Verification items for the finished model (mm, model axes). A direction names the side the tool comes from. Give positions to 0.01 mm unless a question says otherwise; leave off trailing zeros. Loops run counter-clockwise (first coordinate to the right, second up) from the corner with the lowest first, then second, coordinate; pieces in that order, holes last. Notation, with made-up numbers: M 83.25,61 L 133.25,61 A8 cw 133.25,65 Z; hole C 81.25,69.5 d1. An arc over 180 degrees is marked long. Use CSV: the item, a comma, the result in double quotes.
Autodesk Fusion 360 part; units mm, degrees
sketch "Sketch1" plane through (0, 0, 0) normal (0, 0, 1) x (1, 0, 0)
  line L0 (-38.1, 0) -> (38.1, 0)
  line L1 (-9.525, 0) -> (9.525, 0)
  line L2 (9.525, 0) -> (9.525, 69.85)
  line L3 (9.525, 69.85) -> (-9.525, 69.85)
  line L4 (-9.525, 69.85) -> (-9.525, 0)
  line L5 (-38.1, 0) -> (-38.1, 3.175)
  line L6 (-38.1, 3.175) -> (38.1, 3.175)
  line L7 (38.1, 3.175) -> (38.1, 0)
  circle A0 centre (-25.4, 19.05) radius 15.875
  circle A1 centre (25.4, 19.05) radius 15.875
  line L8 (-9.525, 44.45) -> (9.525, 44.45)
  line L9 (-5.715, 69.85) -> (-5.715, 44.45)
  line L10 (-1.905, 69.85) -> (-1.905, 44.45)
  line L11 (1.905, 69.85) -> (1.905, 44.45)
  line L12 (5.715, 69.85) -> (5.715, 44.45)
  dimension "d2" = 19.05
  dimension "d3" = 9.525
  dimension "d4" = 3.175
  dimension "d5" = 76.2
  dimension "d6" = 31.75
  dimension "d7" = 31.75
  dimension "d17" = 69.85
  dimension "d18" = 3.175
  dimension "d28" = 25.4
  dimension "d29" = 3.81
  dimension "d30" = 3.81
  dimension "d31" = 3.81
  dimension "d32" = 3.81
extrude "Extrude1" add sketch "Sketch1" along normal blind 63.5 contours L0 L4 L5 L6 | L0 L1 L2 L4 L6 | L0 L2 L6 L7 | L4 L6 A0 | L2 L4 L6 L8 | L2 L6 A1 | L3 L4 L8 L9 | L2 L3 L8 L12 | L3 L8 L9 L10 | L3 L8 L11 L12 | L3 L8 L10 L11 makes body 1
sketch "Sketch3" plane through (0, 0, 0) normal (1, 0, 0) x (0, 0, -1)
  line L0 (0, 0) -> (-63.5, 0)
  line L1 (-63.5, 0) -> (-63.5, 69.85)
  line L2 (-63.5, 69.85) -> (0, 69.85)
  line L3 (0, 69.85) -> (0, 0)
  line L4 (-63.5, 3.175) -> (0, 3.175)
  line L5 (-19.05, 69.85) -> (-19.05, 0)
  line L6 (0, 3.175) -> (0, 0)
  line L7 (-9.525, 69.85) -> (-9.525, 0)
  line L8 (-28.575, 69.85) -> (-28.575, 0)
  circle A0 centre (-19.05, 60.325) radius 9.525
  arc A1 (-9.525, 13.9553) -> (0, 3.175) centre (0, 12.7731) ccw
  arc A2 (-41.5769, 3.175) -> (-28.575, 16.6144) centre (-41.5769, 16.184) ccw
  circle A3 centre (-19.05, 60.325) radius 2.54
  circle A4 centre (-19.05, 60.325) radius 2.032
  dimension "d15" = 63.5
  dimension "d16" = 69.85
  dimension "d19" = 3.175
  dimension "d20" = 19.05
  dimension "d21" = 9.525
  dimension "d22" = 9.525
  dimension "d23" = 19.05
  dimension "d25" = 5.08
  dimension "d35" = 4.064
extrude "Extrude2" cut sketch "Sketch3" along normal mid plane 81.28 contours L2 L3 L7 A1 | L2 L7 A0 | L2 L8 A0 | L1 L2 L4 L8 A2 | L5 A3 A4 | L5 A3 A4 | L5 A4 | L5 A4 bodies 1
extrude "Extrude3" cut sketch "Sketch1" along normal blind 33.02 contours L3 L8 L9 L10 | L3 L8 L11 L12 bodies 1
extrude "Extrude4" add sketch "Sketch3" along normal blind -9.525 and the other way blind 5.715 contours L5 A3 A4 | L5 A3 A4 bodies 1
copy_body "Body->Comp1" bodies 1 removing the originals makes body 2 in component "Base"
component "Base" placed x (1, 0, 0) y (0, 1, 0) z (0, 0, 1) at (0, 0, 0)
(1) Section check B-B on z = 19.05. Count the separate pieces of the cut face and the enclosed holes in it, plus the area to 3 significant figures.
Calculated:
separate pieces,"4"
enclosed holes,"0"
area,"1,370 mm²"
(2) Scan lines: L1, parallel to X at y = 44.5, z = 27 (3 decimals); L2, parallel to Y at x = -0.9, z = 19.05 (3 decimals); L3, parallel to Y at x = -8, z = 19. Record each from-to range of solid material in increasing order. Write a range as from..to.
Calculated:
L1,"x = -9.525..-5.715, -1.905..1.905, 5.715..9.525"
L2,"y = 0..57.785, 62.865..69.85"
L3,"y = 0..58.29, 62.36..69.85"
(3) Section check A-A on y = 51. Record the cut outline in (x, z) (3 decimals).
Calculated:
outline,"M -9.525,9.525 L -5.715,9.525 L -5.715,28.575 L -9.525,28.575 Z; M -1.905,9.525 L 1.905,9.525 L 1.905,28.575 L -1.905,28.575 Z; M 5.715,9.525 L 9.525,9.525 L 9.525,28.575 L 5.715,28.575 Z"
(4) Depth check by flat-ended pin: pin 1 Ø9.5 at (y, z) = (61, 22) entering from +X (3 decimals); pin 2 Ø9.5 at (y, z) = (57, 19.5) entering from -X (3 decimals); pin 3 Ø4 at (x, z) = (3.5, 21) entering from +Y. Enter the tip coordinate at first touch or a pass-through.
Calculated:
pin 1,"stops at x = 9.525"
pin 2,"stops at x = -9.525"
pin 3,"stops at y = 69.82"
(5) Mould release check, pull along Z, two halves, no side actions. Record for faces 6 (the flat face through (38.1, 2, 31)), 7 (the flat face through (-1, 2, 63.5)), 8 (the cylindrical face through (7.593, 57.807, 19.381)): released by +Z, released by -Z, zero draft, split by the parting line, or undercut.
Calculated:
face 6,"zero draft"
face 7,"released by +Z"
face 8,"undercut"
(6) Section check D-D on z = 5. Record the cut outline in (x, y) (3 decimals).
Calculated:
outline,"M -38.1,0 L 38.1,0 L 38.1,3.175 L 25.4,3.175 A15.875 cw 18.87,4.58 L -18.87,4.58 A15.875 cw -25.4,3.175 L -38.1,3.175 Z"
(7) Section check C-C on x = -20. Record the cut outline in (y, z) (3 decimals).
Calculated:
outline,"M 0,0 L 3.175,0 A9.598 cw 4.122,4.156 L 4.122,36.705 A13.009 cw 3.175,41.577 L 3.175,63.5 L 0,63.5 Z"
(8) Tool access check on faces 1 (the cylindrical face through (-0.027, 57.807, 19.381)), 2 (the flat face through (-9.525, 45, 19)), 3 (the flat face through (5.715, 57, 19)), 4 (the flat face through (9.525, 44, 19)), 5 (the flat face through (0, 33, 28.575)). Record the directions out of +Z, -Z, +X, -X, +Y, -Y that give a thin tool (end or side, any length) a straight path to the whole face; none if there is none.
Calculated:
face 1,"+X"
face 2,"+Z, -Z, -X, +Y"
face 3,"+Z, -Z, +Y"
face 4,"+Z, -Z, +X, +Y"
face 5,"+Z, +X, -X, +Y"
